from build123d import *

# Parameters (mm, degrees)
SKETCH_1_W          = 147
SKETCH_1_H          = 70
EXTRUDE_1_DEPTH     = 2
SKETCH_3_W          = 147
SKETCH_3_H          = 3
CUT_EXTRUDE_1_DEPTH = 82.432487375
SKETCH_5_R          = 2
CUT_EXTRUDE_3_DEPTH = 10
SKETCH_6_R          = 1.6
CUT_EXTRUDE_4_DEPTH = 10
SKETCH_7_W          = 6
SKETCH_7_H          = 48.5
SKETCH_7_H_2        = 50
CUT_EXTRUDE_5_DEPTH = 10
FILLET_1_R          = 3
SKETCH_8_W          = 26
SKETCH_8_H          = 5.5
CUT_EXTRUDE_6_DEPTH = 82.432487375
FILLET_2_R          = 2.5


with BuildPart() as part:
    # 草图1 → 凸台-拉伸1 (new body)
    with BuildSketch(Plane(origin=(0, 0, 0), x_dir=(1, 0, 0), z_dir=(0, 1, 0))):
        Rectangle(SKETCH_1_W, SKETCH_1_H)
    extrude(amount=EXTRUDE_1_DEPTH)

    # 草图3 → 切除-拉伸1 (cut, through all)
    with BuildSketch(Plane(origin=(0, 2, 0), x_dir=(1, 0, 0), z_dir=(0, 1, 0))):
        with Locations((0, 33.5)):
            Rectangle(SKETCH_3_W, SKETCH_3_H)
    extrude(amount=-CUT_EXTRUDE_1_DEPTH, mode=Mode.SUBTRACT)

    # 草图5 → 切除-拉伸3 (cut)
    with BuildSketch(Plane(origin=(0, 2, 0), x_dir=(1, 0, 0), z_dir=(0, 1, 0))):
        with Locations(Location((-8, -29, 0), (0, 0, 270))):
            Circle(SKETCH_5_R)
        with Locations(Location((8, -29, 0), (0, 0, 270))):
            Circle(SKETCH_5_R)
    extrude(amount=-CUT_EXTRUDE_3_DEPTH, mode=Mode.SUBTRACT)

    # 草图6 → 切除-拉伸4 (cut)
    with BuildSketch(Plane(origin=(0, 2, 0), x_dir=(1, 0, 0), z_dir=(0, 1, 0))):
        with Locations(Location((-70.5, 10, 0), (0, 0, 270))):
            Circle(SKETCH_6_R)
        with Locations(Location((70.5, 10, 0), (0, 0, 270))):
            Circle(SKETCH_6_R)
    extrude(amount=-CUT_EXTRUDE_4_DEPTH, mode=Mode.SUBTRACT)

    # 草图7 → 切除-拉伸5 (cut)
    with BuildSketch(Plane(origin=(0, 2, 0), x_dir=(1, 0, 0), z_dir=(0, 1, 0))):
        with Locations((12, -0.75)):
            Rectangle(SKETCH_7_W, SKETCH_7_H)
        with Locations((0, -1.5)):
            Rectangle(SKETCH_7_W, SKETCH_7_H_2)
        with Locations((24, -1.5)):
            Rectangle(SKETCH_7_W, SKETCH_7_H_2)
        with Locations((36, -1.5)):
            Rectangle(SKETCH_7_W, SKETCH_7_H_2)
        with Locations((48, -1.5)):
            Rectangle(SKETCH_7_W, SKETCH_7_H_2)
        with Locations((60, -1.5)):
            Rectangle(SKETCH_7_W, SKETCH_7_H_2)
        with Locations((-12, -0.75)):
            Rectangle(SKETCH_7_W, SKETCH_7_H)
        with Locations((-24, -1.5)):
            Rectangle(SKETCH_7_W, SKETCH_7_H_2)
        with Locations((-36, -1.5)):
            Rectangle(SKETCH_7_W, SKETCH_7_H_2)
        with Locations((-48, -1.5)):
            Rectangle(SKETCH_7_W, SKETCH_7_H_2)
        with Locations((-60, -1.5)):
            Rectangle(SKETCH_7_W, SKETCH_7_H_2)
    extrude(amount=-CUT_EXTRUDE_5_DEPTH, mode=Mode.SUBTRACT)

    # 圆角1
    fillet_1_edges = [part.edges().sort_by_distance(p)[0] for p in [
        (-63, 1, -23.5),
        (-57, 1, -23.5),
        (-57, 1, 26.5),
        (-63, 1, 26.5),
        (-27, 1, -23.5),
        (-39, 1, -23.5),
        (-51, 1, -23.5),
        (-3, 1, -23.5),
        (-15, 1, -23.5),
        (9, 1, -23.5),
        (33, 1, -23.5),
        (21, 1, -23.5),
        (45, 1, -23.5),
        (57, 1, -23.5),
        (63, 1, -23.5),
        (51, 1, -23.5),
        (39, 1, -23.5),
        (27, 1, -23.5),
        (15, 1, -23.5),
        (3, 1, -23.5),
        (-9, 1, -23.5),
        (-21, 1, -23.5),
        (-33, 1, -23.5),
        (-45, 1, -23.5),
        (-45, 1, 26.5),
        (-33, 1, 26.5),
        (-21, 1, 26.5),
        (3, 1, 26.5),
        (27, 1, 26.5),
        (39, 1, 26.5),
        (51, 1, 26.5),
        (63, 1, 26.5),
        (21, 1, 26.5),
        (33, 1, 26.5),
        (45, 1, 26.5),
        (57, 1, 26.5),
        (-3, 1, 26.5),
        (-27, 1, 26.5),
        (-39, 1, 26.5),
        (-51, 1, 26.5),
        (15, 1, 25),
        (9, 1, 25),
        (-15, 1, 25),
        (-9, 1, 25),
    ]]
    fillet(fillet_1_edges, radius=FILLET_1_R - 0.0001)  # a hair under: the kernel refuses the full size

    # 草图8 → 切除-拉伸6 (cut, through all)
    with BuildSketch(Plane(origin=(0, 2, 0), x_dir=(1, 0, 0), z_dir=(0, 1, 0))):
        with Locations((0, -35)):
            Rectangle(SKETCH_8_W, SKETCH_8_H)
    extrude(amount=-CUT_EXTRUDE_6_DEPTH, mode=Mode.SUBTRACT)

    # 圆角2
    fillet_2_edges = [part.edges().sort_by_distance(p)[0] for p in [
        (13, 1, 35),
        (-13, 1, 35),
    ]]
    fillet(fillet_2_edges, radius=FILLET_2_R)


solid = part.part
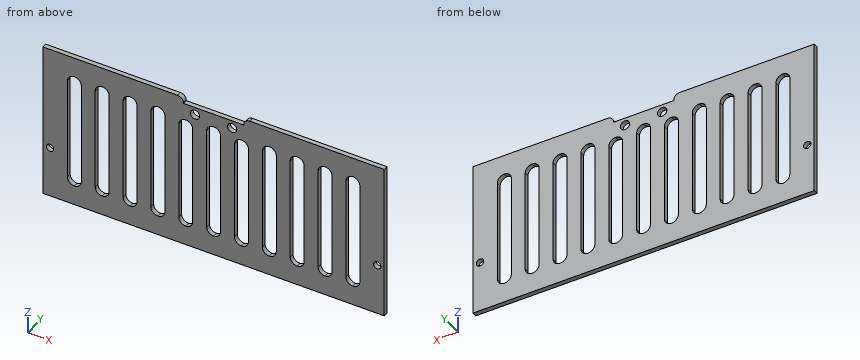
Build history of the part. All positions in model axes, mm. Round coordinates to 2 decimals unless told otherwise and drop trailing zeros. Write each loop counter-clockwise with the first axis right and the second up, starting at its lowest first coordinate (ties: lowest second). Pieces come first, ordered by that corner, then holes. Notation, with made-up numbers: (10.5, 35.25) - (64.5, 35.25) arc R25 cw to (64.5, 47.25) - close; hole circle Ø10 at (19.5, -38). An arc over 180 degrees is marked (long way). One line per question, with ' | ' between items.
1. Band-saw the part on A-A, the plane z = 29. Write the cut outline in (x, y), and give its area (3 significant figures).
Results are:
outline: (-73.5, 0) - (-10, 0) - (-10, 2) - (-73.5, 2) - close; (-6, 0) - (6, 0) - (6, 2) - (-6, 2) - close; (10, 0) - (73.5, 0) - (73.5, 2) - (10, 2) - close | area: 278 mm^2
2. Band-saw the part on B-B, the plane x = 70.5. Write the cut outline in (y, z), and give its area (3 significant figures).
Results are:
outline: (0, -32) - (2, -32) - (2, -11.6) - (0, -11.6) - close; (0, -8.4) - (2, -8.4) - (2, 35) - (0, 35) - close | area: 128 mm^2
3. Drill centre lines: line 1 along X through (y, z) = (0.5, 29); line 2 along Z through (x, y) = (-70.5, 0.65); line 3 along Z through (x, y) = (-24, 1.1). Where is each one in solid material? Low to high. Write a range as from..to.
Results are:
line 1: -73.5..-10, -6..6, 10..73.5 | line 2: -32..-11.6, -8.4..35 | line 3: -32..-23.5, 26.5..35
4. Band-saw the part on C-C, the plane z = -10. Give the number of separate pieces and of enclosed holes in the cut face, and give its area (3 significant figures).
Results are:
separate pieces: 14 | enclosed holes: 0 | area: 149 mm^2
